CAD build for the part. Positions are in the model's coordinates, mm. A direction names the side the tool comes from. Round coordinates to 2 decimals unless told otherwise and drop trailing zeros. Write each loop counter-clockwise with the first axis right and the second up, starting at its lowest first coordinate (ties: lowest second). Pieces come first, ordered by that corner, then holes. Notation, with made-up numbers: (7.5, -23.75) - (22.5, -23.75) arc R26 cw to (22.5, 3.25) - close; hole circle Ø1 at (61, 84). An arc over 180 degrees is marked (long way). Put each result on its own line as item: value. Start each with the question number.
Item 1: Drill centre lines: line 1 (Y direction, x = 23, z = 20); line 2 (Z direction, x = -9.5, y = -48); line 3 (X direction, y = -47, z = 40). Where is each one in solid material? Low to high. Write a range as from..to.
Item 2: Pin check, flat tips, straight feed: pin 1 Ø0.8 at (y, z) = (-8, -1) entering from +X; pin 2 Ø5 at (x, y) = (-51, -3.5) entering from -Z; pin 3 Ø0.5 at (y, z) = (4, -0.5) entering from -X. Stop position of each tip, or through.
Item 3: 3-axis set-ups, long thin cutter, end or side, ignore diameter. For faces 5 (the cylindrical face through (-60.202, 38.559, -0.805)), 6 (the cylindrical face through (-73.67, -38.41, -0.8)), 7 (the cylindrical face through (79.728, -55.916, 28.722)): which of +Z, -Z, +X, -X, +Y, -Y reach the whole face in a straight line?
Item 4: Cut at B-B (x = -74). Give the cut face in (y, z).
Item 5: Mould opens along X. For faces 1 (the cylindrical face through (60.054, -38.411, -0.805)), 2 (the flat face through (77, -63, 34)), 3 (the cylindrical face through (-85.789, 0.7, 43.205)), 4 (the cylindrical face through (-60.202, -38.559, -0.805)) say: released by +X, released by -X, zero draft, split by the parting line, or undercut.
Item 6: Cut at C-C (z = 23.5). Give the cut face in (x, y), and give its area (3 significant figures).
Item 7: Cut at D-D (y = -10). Give the cut face in (x, z), and give its area (3 significant figures).
Item 8: Cut at A-A (y = -44.5). Give the cut face in (x, z).
```python
from build123d import *

# Parameters (mm, degrees)
F0_W     = 175
F0_H     = 100
F1_DEPTH = 45.0088
F2_R     = 6.35
F3_DEPTH = 13
F4_SIZE  = 1
F5_R     = 6
F6_W     = 19.05
F6_H     = 82.55
F7_DEPTH = 1.5875
F8_R     = 9.52499


# Not quite as in the source:
# - a fillet or chamfer is up to 0.001 mm smaller than in the source, because OpenCascade refuses the exact size
# - a length typed as a fraction of an inch, garbled in the dataset ("3 / 203.2 mm" for 3/8 in), is restored
# - a pattern or mirror of a feature is missing from the dataset's text; its kind, count and spacing are read off the source's solid


with BuildPart() as f1:
    # F0 (on Top) → F1 (new body)
    with BuildSketch(Plane.XY):
        Rectangle(F0_W, F0_H)
    extrude(amount=F1_DEPTH)

    # F2 (on face) → F3 (join)
    with BuildSketch(Plane.XZ.offset(50)):
        with Locations((76.7980482321, 34.3557204665)):
            Circle(F2_R)
    extrude(amount=F3_DEPTH)

    # F4
    f4_edges = [f1.edges().sort_by_distance(p)[0] for p in [
        (70.448048, -63, 34.35572),
    ]]
    chamfer(f4_edges, length=F4_SIZE)

    # F5
    f5_edges = [f1.edges().sort_by_distance(p)[0] for p in [
        (-87.5, 0, 45.0088),
        (87.5, 0, 45.0088),
        (87.5, 0, 0),
        (-87.5, 0, 0),
    ]]
    fillet(f5_edges, radius=F5_R)

    # F6 (on face) → F7 (join)
    with BuildSketch(Plane(origin=(0, 0, 0), x_dir=(1, 0, 0), z_dir=(0, 0, -1))):
        with Locations((-66.8625, 0)):
            Rectangle(F6_W, F6_H)
    f7 = extrude(amount=F7_DEPTH)

    # F7_copies: F7 across plane
    add(f7.mirror(Plane(origin=(0, 0, 0), x_dir=(0, 0, 1), z_dir=(1, 0, 0))))

    # F8 (radius 9.525 in the source; OpenCascade refuses exactly that, so slightly less here)
    f8_edges = [f1.edges().sort_by_distance(p)[0] for p in [
        (-76.3875, -41.275, -0.79375),
        (-57.3375, -41.275, -0.79375),
        (-76.3875, 41.275, -0.79375),
        (-57.3375, 41.275, -0.79375),
        (76.3875, -41.275, -0.79375),
        (76.3875, 41.275, -0.79375),
        (57.3375, 41.275, -0.79375),
        (57.3375, -41.275, -0.79375),
    ]]
    fillet(f8_edges, radius=F8_R)


solid = f1.part
```
Output values:
1. line 1: -50..50
1. line 2: 0..45.01
1. line 3: -87.42..87.42
2. pin 1: x = 76.39
2. pin 2: z = 0
2. pin 3: x = -76.39
3. face 5: -Z, +Y
3. face 6: -Z, -X, -Y
3. face 7: -Y
4. outline: (-50, 0) - (-38.06, 0) - (-38.06, -1.59) - (38.06, -1.59) - (38.06, 0) - (50, 0) - (50, 45.01) - (-50, 45.01) - close
5. face 1: undercut
5. face 2: zero draft
5. face 3: released by -X
5. face 4: undercut
6. outline: (-87.5, -50) - (87.5, -50) - (87.5, 50) - (-87.5, 50) - close
6. area: 17,500 mm2
7. outline: (-87.5, 6) arc R6 ccw to (-81.5, 0) - (-76.39, 0) - (-76.39, -1.59) - (-57.34, -1.59) - (-57.34, 0) - (57.34, 0) - (57.34, -1.59) - (76.39, -1.59) - (76.39, 0) - (81.5, 0) arc R6 ccw to (87.5, 6) - (87.5, 39.01) arc R6 ccw to (81.5, 45.01) - (-81.5, 45.01) arc R6 ccw to (-87.5, 39.01) - close
7. area: 7,910 mm2
8. outline: (-87.5, 6) arc R6 ccw to (-81.5, 0) - (81.5, 0) arc R6 ccw to (87.5, 6) - (87.5, 39.01) arc R6 ccw to (81.5, 45.01) - (-81.5, 45.01) arc R6 ccw to (-87.5, 39.01) - close
